from build123d import *

# Parameters (mm, degrees)
SKETCH2_W                 = 37.5
SKETCH2_H                 = 95
BOSS_EXTRUDE1_DEPTH       = 15
SKETCH3_W                 = 30
SKETCH3_H                 = 42
CUT_EXTRUDE1_DEPTH        = 10
SKETCH5_R                 = 8.5
SKETCH5_W                 = 30
SKETCH5_H                 = 6.6
CUT_EXTRUDE2_DEPTH        = 50
CUT_EXTRUDE3_DEPTH        = 10
SKETCH7_W                 = 6.5
SKETCH7_H                 = 9
CUT_EXTRUDE4_DEPTH        = 3.75
SKETCH8_W                 = 12.75
SKETCH8_H                 = 3
BOSS_EXTRUDE2_DEPTH       = 10
F_2_5MM_DOWEL_HOLE2_D     = 3.75
SKETCH14_W                = 37.5
SKETCH14_H                = 15
BOSS_EXTRUDE3_DEPTH       = 14.5
CUT_EXTRUDE5_DEPTH        = 11.1125
SKETCH16_W                = 8.89
SKETCH16_H                = 8.8125
BOSS_EXTRUDE4_DEPTH       = 1
SKETCH17_W                = 3.75
SKETCH17_H                = 10
BOSS_EXTRUDE5_DEPTH       = 10
F_2_5MM_DOWEL_HOLE3_D     = 3.75
SKETCH24_W                = 37.5
SKETCH24_H                = 4.3875
BOSS_EXTRUDE7_DEPTH       = 87.5
BOSS_EXTRUDE8_DEPTH       = 10
SKETCH26_W                = 37.5
SKETCH26_H                = 9.690281336
BOSS_EXTRUDE9_DEPTH       = 7.5
SKETCH27_W                = 20.05
SKETCH27_H                = 6.4
CUT_EXTRUDE6_DEPTH        = 14.6
FILLET2_R                 = 2
F_2_5MM_DOWEL_HOLE4_D     = 5.5
F_2_5MM_DOWEL_HOLE4_DEPTH = 5
F_2_5MM_DOWEL_HOLE4_TIP   = 1.652366702
SKETCH31_W                = 4.284862737
SKETCH31_H                = 6.4
CUT_EXTRUDE7_DEPTH        = 112.002252229
CUT_EXTRUDE8_DEPTH        = 1.5


with BuildPart() as part:
    # Sketch2 → Boss-Extrude1 (new body)
    with BuildSketch(Plane(origin=(0, 0, 0), x_dir=(1, 0, 0), z_dir=(0, 1, 0))):
        with Locations((18.75, 47.5)):
            Rectangle(SKETCH2_W, SKETCH2_H)
    extrude(amount=BOSS_EXTRUDE1_DEPTH)

    # Sketch3 → Cut-Extrude1 (cut)
    with BuildSketch(Plane(origin=(0, 15, 0), x_dir=(1, 0, 0), z_dir=(0, 1, 0))):
        with Locations((18.75, 21)):
            Rectangle(SKETCH3_W, SKETCH3_H)
    extrude(amount=-CUT_EXTRUDE1_DEPTH, mode=Mode.SUBTRACT)

    # Sketch5 → Cut-Extrude2 (cut)
    with BuildSketch(Plane.XY.offset(-42)):
        with Locations((18.75, 15)):
            Circle(SKETCH5_R)
        with Locations((18.75, 11.7)):
            Rectangle(SKETCH5_W, SKETCH5_H)
    extrude(amount=-CUT_EXTRUDE2_DEPTH, mode=Mode.SUBTRACT)

    # Sketch6 → Cut-Extrude3 (cut)
    with BuildSketch(Plane(origin=(0, 0, -95), x_dir=(-1, 0, 0), z_dir=(0, 0, -1))):
        with BuildLine():
            Line((-21.75, 15), (-15.75, 15))
            ThreePointArc((-15.75, 15), (-18.75, 12), (-21.75, 15))
        make_face()
    extrude(amount=-CUT_EXTRUDE3_DEPTH, mode=Mode.SUBTRACT)

    # Sketch7 → Cut-Extrude4 (cut)
    with BuildSketch(Plane.ZY.offset(-37.5)):
        with Locations((-15.25, 10.5)):
            Rectangle(SKETCH7_W, SKETCH7_H)
    extrude(amount=CUT_EXTRUDE4_DEPTH, mode=Mode.SUBTRACT)

    # Sketch8 → Boss-Extrude2 (add)
    with BuildSketch(Plane(origin=(0, 15, 0), x_dir=(1, 0, 0), z_dir=(0, 1, 0))):
        with Locations((6.375, 93.5)):
            Rectangle(SKETCH8_W, SKETCH8_H)
    boss_extrude2 = extrude(amount=BOSS_EXTRUDE2_DEPTH)

    # Mirror1: Boss-Extrude2 across plane
    add(boss_extrude2.mirror(Plane.ZY.offset(-18.75)))

    # Ø2.5mm Dowel Hole2 (through all)
    with Locations(Plane(origin=(37.5, 0, 0), x_dir=(0, 0, -1), z_dir=(1, 0, 0))):
        with Locations((5.25, 10)):
            Hole(F_2_5MM_DOWEL_HOLE2_D / 2)

    # Sketch14 → Boss-Extrude3 (add)
    with BuildSketch(Plane.XZ):
        with Locations((18.75, -95)):
            Rectangle(SKETCH14_W, SKETCH14_H)
    extrude(amount=BOSS_EXTRUDE3_DEPTH)

    # Sketch15 → Cut-Extrude5 (cut)
    with BuildSketch(Plane.XZ.offset(14.5)):
        Polygon((16.143541, -102.5), (16.143541, -100), (12.003125, -100), (12.003125, -96.3125), (14.305, -96.3125), (14.305, -87.5), (23.195, -87.5), (23.195, -96.3125), (25.496875, -96.3125), (25.496875, -100), (21.356459, -100), (21.356459, -102.5), align=None)
    extrude(amount=-CUT_EXTRUDE5_DEPTH, mode=Mode.SUBTRACT)

    # Sketch16 → Boss-Extrude4 (add)
    with BuildSketch(Plane.XZ.offset(3.3875)):
        with Locations((18.75, -91.90625)):
            Rectangle(SKETCH16_W, SKETCH16_H)
    extrude(amount=BOSS_EXTRUDE4_DEPTH)

    # Sketch17 → Boss-Extrude5 (add)
    with BuildSketch(Plane(origin=(0, 15, 0), x_dir=(1, 0, 0), z_dir=(0, 1, 0))):
        with Locations((1.875, 87)):
            Rectangle(SKETCH17_W, SKETCH17_H)
        with Locations((35.625, 87)):
            Rectangle(SKETCH17_W, SKETCH17_H)
    extrude(amount=BOSS_EXTRUDE5_DEPTH)

    # Ø2.5mm Dowel Hole3 (through all)
    with Locations(Plane(origin=(37.5, 0, 0), x_dir=(0, 0, -1), z_dir=(1, 0, 0))):
        with Locations((87.486504599, 20.104293775)):
            Hole(F_2_5MM_DOWEL_HOLE3_D / 2)

    # Sketch24 → Boss-Extrude7 (add)
    with BuildSketch(Plane.XY.offset(-87.5)):
        with Locations((18.75, -2.19375)):
            Rectangle(SKETCH24_W, SKETCH24_H)
    extrude(amount=BOSS_EXTRUDE7_DEPTH)

    # Sketch25 → Boss-Extrude8 (add)
    with BuildSketch(Plane.XY):
        with BuildLine():
            Line((37.5, -4.3875), (18.75, -4.3875))
            ThreePointArc((18.75, -4.3875), (21.578427125, -5.559072875), (22.75, -8.3875))
            Line((22.75, -8.3875), (37.5, -8.3875))
            Line((37.5, -8.3875), (37.5, -4.3875))
        make_face()
        with BuildLine():
            Line((18.75, -4.3875), (0, -4.3875))
            Line((0, -4.3875), (0, -8.3875))
            Line((0, -8.3875), (14.75, -8.3875))
            ThreePointArc((14.75, -8.3875), (15.921572875, -5.559072875), (18.75, -4.3875))
        make_face()
    extrude(amount=-BOSS_EXTRUDE8_DEPTH)

    # Sketch26 → Boss-Extrude9 (add)
    with BuildSketch(Plane(origin=(0, 0, -95), x_dir=(-1, 0, 0), z_dir=(0, 0, -1))):
        with Locations((-18.75, 4.845140668)):
            Rectangle(SKETCH26_W, SKETCH26_H)
    extrude(amount=BOSS_EXTRUDE9_DEPTH)

    # Sketch27 → Cut-Extrude6 (cut)
    with BuildSketch(Plane(origin=(0, 0, -102.5), x_dir=(-1, 0, 0), z_dir=(0, 0, -1))):
        with Locations((-13.025, 2.990281336)):
            Rectangle(SKETCH27_W, SKETCH27_H)
    extrude(amount=-CUT_EXTRUDE6_DEPTH, mode=Mode.SUBTRACT)

    # Fillet2
    fillet2_edges = [part.edges().sort_by_distance(p)[0] for p in [
        (0, -9.44375, -87.5),
        (0, -2.404859332, -102.5),
        (37.5, -2.404859332, -102.5),
        (37.5, -9.44375, -87.5),
        (0, -14.5, -95),
        (8.0717705, -14.5, -102.5),
        (37.5, -14.5, -95),
        (30.3475, -14.5, -87.5),
        (29.4282295, -14.5, -102.5),
        (7.1525, -14.5, -87.5),
        (37.5, -4.3875, -48.75),
        (37.5, -6.3875, -10),
        (0, -4.3875, -48.75),
        (0, -6.3875, -10),
        (0, 17.345140668, -95),
        (37.5, 17.345140668, -95),
        (37.5, 3.30625, 0),
        (0, 3.30625, 0),
    ]]
    fillet(fillet2_edges, radius=FILLET2_R)

    # Ø2.5mm Dowel Hole4
    with Locations(Plane(origin=(0, -8.3875, 0), x_dir=(-1, 0, 0), z_dir=(0, -1, 0))):
        with Locations((-32.5, 5), (-5, 5)):
            Hole(F_2_5MM_DOWEL_HOLE4_D / 2, depth=F_2_5MM_DOWEL_HOLE4_DEPTH)
            with Locations((0, 0, -(F_2_5MM_DOWEL_HOLE4_DEPTH + F_2_5MM_DOWEL_HOLE4_TIP / 2))):  # 118° drill point
                Cone(0, F_2_5MM_DOWEL_HOLE4_D / 2, F_2_5MM_DOWEL_HOLE4_TIP, mode=Mode.SUBTRACT)

    # Sketch31 → Cut-Extrude7 (cut, through all)
    with BuildSketch(Plane(origin=(3, 0, 0), x_dir=(0, 0, -1), z_dir=(1, 0, 0))):
        with Locations((90.042431369, 2.990281336)):
            Rectangle(SKETCH31_W, SKETCH31_H)
    extrude(amount=-CUT_EXTRUDE7_DEPTH, mode=Mode.SUBTRACT)

    # Sketch32 → Cut-Extrude8 (cut)
    with BuildSketch(Plane.XZ.offset(4.3875)):
        Polygon((32.662211036, -66.731402862), (32.662211036, -60.842760163), (31.314060446, -61.257991767), (31.314060446, -51.061409973), (31.181038698, -49.082813371), (30.740043615, -47.651015368), (30.272932489, -46.702611031), (29.343491661, -45.825186496), (28.166570354, -45.289551545), (26.913013893, -45.172232341), (25.487931235, -45.415918592), (23.663222713, -46.115147592), (22.123128119, -47.024353691), (21.210078183, -47.821011367), (20.018893116, -49.082813371), (18.887507594, -51.061409973), (18.257769049, -52.911736478), (17.912229988, -55.231688956), (19.282356905, -54.7066558), (19.282356905, -61.531664738), (17.863237505, -62.075471832), (17.863237505, -66.360306951), (16.408711909, -66.917681713), (16.408711909, -72.685258984), (23.193470428, -70.305264788), (23.193470428, -54.347624256), (23.331002369, -53.424233522), (23.59042172, -52.661995758), (24.115625328, -52.105656542), (24.950101738, -51.812934405), (25.728287005, -52.077781315), (25.967613662, -52.760040784), (25.967613662, -69.19073609), align=None)
        Polygon((18.887507594, -61.257991767), (18.887507594, -55.376949047), (17.389382, -55.927301794), (17.389382, -43.806150983), (18.887507594, -43.255798236), (18.887507594, -37.448382085), (13.405832614, -39.371273607), (11.177740444, -40.341723555), (10.100640592, -40.98328383), (8.936720005, -41.849530032), (7.790955921, -42.951413953), (6.783486907, -44.128073894), (6.081538262, -45.289551545), (5.270405037, -47.097284534), (4.808853701, -48.478793464), (4.295716054, -50.413974213), (4.021830569, -53.238519595), (4.021830569, -56.833755888), (4.295716054, -58.862358442), (4.808853701, -60.527748098), (5.381572286, -61.842674021), (6.348688627, -62.848303696), (7.790955921, -63.886150712), (9.142953346, -64.244649926), (10.639190518, -64.244649926), (11.974170787, -63.886150712), align=None)
        Polygon((12.135932336, -57.848057165), (12.135932336, -45.679668485), (11.306680653, -46.296837843), (10.540601176, -47.191570107), (9.999416807, -48.284787608), (9.642235274, -49.631815705), (9.392627445, -51.131802286), (9.330267236, -52.833612335), (9.392627445, -54.227691449), (9.569214099, -55.535625441), (9.82082604, -56.47257862), (10.338657712, -57.470582903), (10.923640914, -57.97145187), (11.554307118, -57.97145187), align=None, mode=Mode.SUBTRACT)
    extrude(amount=-CUT_EXTRUDE8_DEPTH, mode=Mode.SUBTRACT)


solid = part.part
Work out the finished part from the listing and answer in its coordinate system (mm). A direction names the side the tool comes from. Give positions to 0.01 mm unless a question says otherwise; leave off trailing zeros. Loops run counter-clockwise (first coordinate to the right, second up) from the corner with the lowest first, then second, coordinate; pieces in that order, holes last. Notation, with made-up numbers: (-39, -36) - (5, -36) arc R29 cw to (5, -7) - close; hole circle Ø4 at (-18.75, 47.5). An arc over 180 degrees is marked (long way). Answer in a Markdown table with one row per item. Add a question column.
Q1. Each of these flat-tipped pins is pushed along its axis until it touches: P1, Ø12, axis at x = 14.5, z = -45.5, coming from the -Y side; P2, Ø10, axis at x = 32.5, z = -13, coming from the -Y side; P3, Ø1.6, axis at y = -4, z = -55.5, coming from the +X side. Where does it stop, or does it pass through?
Q2. The part is cut by section C-C (y = -10.5). Determine the outline of the cut face in (x, z) (1 decimal).
Q3. Consider line 1 along Z through (x, y) = (13.5, -8); line 2 along Z through (x, y) = (32.5, -7.5); line 3 along X through (y, z) = (9.5, -38). Determine where each line is inside the solid, lowest interval first.
Q4. The part is cut by section A-A (y = 16.5). Determine the outline of the cut face in (x, z), and give its area (3 significant figures).
Q5. Determine the mould class of faces 5 (the flat face through (16.185, -3.648, -38.396)), 6 (the flat face through (0, 6, -51)), 7 (the flat face through (2, 15, -42)) for opening direction X: released by +X, released by -X, zero draft, split by the parting line, or undercut.
Q6. The part is cut by section B-B (y = -5.5). State how many separate pieces and enclosed holes the cut face has, and give its area (3 significant figures).
Q7. A tool of negligible diameter and unlimited length cuts with its end or side. For faces 1 (the cylindrical face through (0.601, -3.817, -48.179)), 2 (the flat face through (14, 15, -94)), 3 (the flat face through (21.356, -9, -101)), 4 (the cylindrical face through (36.93, -8.64, -88.1)), from which of +Z, -Z, +X, -X, +Y, -Y can it reach the whole face along a straight path? Write none if from no direction.
Solution:
| question | item | result |
|---|---|---|
| 1 | P1 | stops at y = -4.39 |
| 1 | P2 | stops at y = -8.39 |
| 1 | P3 | stops at x = 37.33 |
| 2 | outline | (0, -100.5) arc R2 ccw to (2, -102.5) - (16.1, -102.5) - (16.1, -100) - (12, -100) - (12, -96.3) - (14.3, -96.3) - (14.3, -87.5) - (2, -87.5) arc R2 ccw to (0, -89.5) - close; (21.4, -102.5) - (35.5, -102.5) arc R2 ccw to (37.5, -100.5) - (37.5, -89.5) arc R2 ccw to (35.5, -87.5) - (23.2, -87.5) - (23.2, -96.3) - (25.5, -96.3) - (25.5, -100) - (21.4, -100) - close |
| 3 | line 1 | z = -102.5 to -100, -96.31 to -87.5, -10 to 0 |
| 3 | line 2 | z = -102.5 to -87.5, -10 to -7.75, -2.25 to 0 |
| 3 | line 3 | x = 0 to 3.75, 33.75 to 37.5 |
| 4 | outline | (0, -93) arc R2 ccw to (2, -95) - (12.75, -95) - (12.75, -92) - (3.75, -92) - (3.75, -82) - (0, -82) - close; (24.75, -95) - (35.5, -95) arc R2 ccw to (37.5, -93) - (37.5, -82) - (33.75, -82) - (33.75, -92) - (24.75, -92) - close |
| 4 | area | 150 mm² |
| 5 | face 5 | undercut |
| 5 | face 6 | released by -X |
| 5 | face 7 | zero draft |
| 6 | separate pieces | 4 |
| 6 | enclosed holes | 2 |
| 6 | area | 687 mm² |
| 7 | face 1 | -X, -Y |
| 7 | face 2 | +Z, -Z, +Y |
| 7 | face 3 | -Z, -Y |
| 7 | face 4 | +X, -Y |
